```python
from build123d import *

# Parameters (mm, degrees)
SKETCH1_R           = 4.7
BOSS_EXTRUDE1_DEPTH = 4
BOSS_EXTRUDE2_DEPTH = 10
CUT_EXTRUDE1_DEPTH  = 3


with BuildPart() as part:
    # Sketch1 → Boss-Extrude1 (new body)
    with BuildSketch(Plane.XY):
        with BuildLine():
            ThreePointArc((-2.35, 13.90278749), (0, -14.1), (2.35, 13.90278749))
            Line((2.35, 13.90278749), (4.585741176, 41.864603012))
            ThreePointArc((4.585741176, 41.864603012), (4.597967377, 43.28721197), (4.408193437, 44.697159337))
            Line((4.408193437, 44.697159337), (2.559360842, 53.589805153))
            ThreePointArc((2.559360842, 53.589805153), (2.402477907, 54.602201264), (2.35, 55.625335767))
            Line((2.35, 55.625335767), (2.35, 65.9))
            Line((2.35, 65.9), (-2.35, 65.9))
            Line((-2.35, 65.9), (-2.35, 55.625335767))
            ThreePointArc((-2.35, 55.625335767), (-2.402477907, 54.602201264), (-2.559360842, 53.589805153))
            Line((-2.559360842, 53.589805153), (-4.408193437, 44.697159337))
            ThreePointArc((-4.408193437, 44.697159337), (-4.597967377, 43.28721197), (-4.585741176, 41.864603012))
            Line((-4.585741176, 41.864603012), (-2.35, 13.90278749))
        make_face()
        Circle(SKETCH1_R, mode=Mode.SUBTRACT)
    extrude(amount=BOSS_EXTRUDE1_DEPTH)

    # Sketch1_3 → Boss-Extrude2 (add)
    with BuildSketch(Plane.XY):
        with BuildLine():
            Line((0, 4.7), (0, 0))
            Line((0, 0), (4.7, 0))
            ThreePointArc((4.7, 0), (3.323401872, 3.323401872), (0, 4.7))
        make_face()
        with BuildLine():
            Line((4.7, 0), (0, 0))
            Line((0, 0), (0, -4.7))
            ThreePointArc((0, -4.7), (3.323401872, -3.323401872), (4.7, 0))
        make_face()
        with BuildLine():
            Line((0, -4.7), (0, 0))
            Line((0, 0), (0, 4.7))
            ThreePointArc((0, 4.7), (-4.7, 0), (0, -4.7))
        make_face()
    extrude(amount=BOSS_EXTRUDE2_DEPTH)

    # Sketch2 → Cut-Extrude1 (cut)
    with BuildSketch(Plane.XY.offset(10)):
        with BuildLine():
            Line((1.7, 1), (1.7, -1))
            ThreePointArc((1.7, -1), (0, -2.7), (-1.7, -1))
            Line((-1.7, -1), (-1.7, 1))
            ThreePointArc((-1.7, 1), (0, 2.7), (1.7, 1))
        make_face()
    extrude(amount=-CUT_EXTRUDE1_DEPTH, mode=Mode.SUBTRACT)


solid = part.part
```
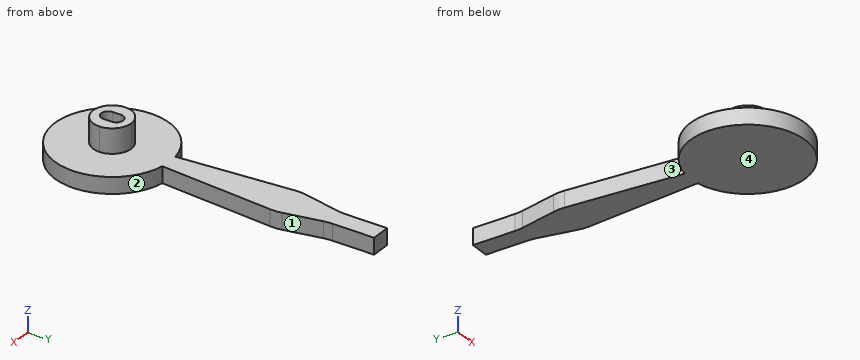
Input: part model. Units: mm. Frame: model coordinates. Face numbers are marked on the shaded views. Coordinates: 2 decimals unless noted, no trailing zeros. Order: outer loops, then holes, each group sorted by start corner. A loop starts at its lowest first (then second) coordinate and runs counter-clockwise, first axis right, second up. Notation, with made-up numbers: (-4, 49.5) - (42, 49.5) arc R29 cw to (42, 69.5) - close; hole circle Ø2 at (-5.5, -28.5). An arc over 180 degrees is marked (long way). Put each result on its own line as item: value.
1. Draft query along X for the marked faces 1, 2, 3 and 4. Return one class per face: pulls with the +X half, pulls with the -X half, needs draft (parallel to the pull), parting line crosses it, or undercut.
Report:
face 1: pulls with the +X half
face 2: parting line crosses it
face 3: pulls with the -X half
face 4: needs draft
2. Cut plane A-A on z = 8.5. Return the cut outline in (x, y).
Report:
outline: circle Ø9.4 at (0, 0); hole (-1.7, -1) arc R1.7 ccw to (1.7, -1) - (1.7, 1) arc R1.7 ccw to (-1.7, 1) - close
3. Cut plane B-B on z = 1.5. Return the cut outline in (x, y), then the cut area to 3 significant figures.
Report:
outline: (-4.59, 41.86) - (-2.35, 13.9) arc R14.1 ccw (long way) to (2.35, 13.9) - (4.59, 41.86) arc R10 ccw to (4.41, 44.7) - (2.56, 53.59) arc R10 cw to (2.35, 55.63) - (2.35, 65.9) - (-2.35, 65.9) - (-2.35, 55.63) arc R10 cw to (-2.56, 53.59) - (-4.41, 44.7) arc R10 ccw to start
area: 964 mm2
4. Cut plane C-C on y = 8. Return the cut outline in (x, z).
Report:
outline: (-11.61, 0) - (11.61, 0) - (11.61, 4) - (-11.61, 4) - close
5. Line query: line 1 along Z through (x, y) = (-2.5, -5.5); line 2 along X through (y, z) = (61.5, 3); line 3 along Y through (x, z) = (0.5, 2.5). Output: solid intervals per line, ascending.
Report:
line 1: z = 0 to 4
line 2: x = -2.35 to 2.35
line 3: y = -14.09 to 65.9
6. Contact query for flat-ended pins moving along their axis: pin 1 Ø6 at (x, y) = (7, 33) entering from +Z; pin 2 Ø3 at (y, z) = (63, 1.5) entering from +X; pin 3 Ø4.5 at (y, z) = (60, 2) entering from -X; pin 4 Ø1 at (y, z) = (0, 9) entering from +X. Output: stop coordinate, or through.
Report:
pin 1: passes through
pin 2: stops at x = 2.35
pin 3: stops at x = -2.35
pin 4: stops at x = 4.7
7. Cut plane D-D on x = 7.75. Return the cut outline in (y, z).
Report:
outline: (-11.78, 0) - (11.78, 0) - (11.78, 4) - (-11.78, 4) - close
